Build history of the part. All positions in model axes, mm. A direction names the side the tool comes from. Round coordinates to 2 decimals unless told otherwise and drop trailing zeros. Loops run counter-clockwise (first coordinate to the right, second up) from the corner with the lowest first, then second, coordinate; pieces in that order, holes last. Notation, with made-up numbers: (86, 80.25) - (96, 80.25) arc R14 ccw to (96, 103.25) - close; hole circle Ø7 at (-30.75, 22). An arc over 180 degrees is marked (long way). One line per question, with ' | ' between items. Start each with the question number.
Autodesk Inventor part; units mm, degrees
ref_plane "YZ Plane" through (0, 0, 0) normal (1, 0, 0) x (0, 1, 0)
ref_plane "XZ Plane" through (0, 0, 0) normal (0, 1, 0) x (-1, 0, 0)
ref_plane "XY Plane" through (0, 0, 0) normal (0, 0, 1) x (1, 0, 0)
sketch "Sketch1" plane through (0, 0, 0) normal (0, 1, 0) x (-1, 0, 0)
  line L0 (22.352, 6.35) -> (-46.355, 6.35)
  line L1 (-46.355, 6.35) -> (-46.355, -6.35)
  line L2 (-46.355, -6.35) -> (22.352, -6.35)
  line L3 (22.352, -6.35) -> (22.352, 6.35)
  line L4 (-2.54, -2.54) -> (2.54, -2.54)
  line L5 (2.54, -2.54) -> (2.54, 2.54)
  line L6 (2.54, 2.54) -> (-2.54, 2.54)
  line L7 (-2.54, 2.54) -> (-2.54, -2.54)
  line L8 (-2.54, -2.54) -> (2.54, 2.54) construction
  line L9 (2.54, -2.54) -> (-2.54, 2.54) construction
  line L10 (-10.16, 2.54) -> (-15.24, 2.54)
  line L11 (-15.24, 2.54) -> (-15.24, -2.54)
  line L12 (-15.24, -2.54) -> (-10.16, -2.54)
  line L13 (-10.16, -2.54) -> (-10.16, 2.54)
  line L14 (-10.16, 2.54) -> (-15.24, -2.54) construction
  line L15 (-15.24, 2.54) -> (-10.16, -2.54) construction
  line L16 (-22.86, 2.54) -> (-27.94, 2.54)
  line L17 (-27.94, 2.54) -> (-27.94, -2.54)
  line L18 (-27.94, -2.54) -> (-22.86, -2.54)
  line L19 (-22.86, -2.54) -> (-22.86, 2.54)
  line L20 (-22.86, 2.54) -> (-27.94, -2.54) construction
  line L21 (-27.94, 2.54) -> (-22.86, -2.54) construction
  point P0 (0, 0)
  point P1 (-12.7, 0)
  point P2 (-25.4, 0)
  dimension "d0" = 68.707
  dimension "d1" = 12.7
  dimension "d2" = 5.08
  dimension "d3" = 5.08
  dimension "d4" = 5.08
  dimension "d5" = 5.08
  dimension "d6" = 12.7
  dimension "d7" = 12.7
  dimension "d8" = 6.35
  dimension "d9" = 22.352
  dimension "d37" = 5.08
  dimension "d38" = 5.08
extrude "Extrusion1" add sketch "Sketch1" along normal blind 2.286
sketch "Sketch2" plane through (0, 2.286, 0) normal (0, 1, 0) x (1, 0, 0)
  line L0 (-22.352, 6.35) -> (-22.352, -6.35)
  circle A0 centre (-16.002, 0) radius 4.191
  point P0 (0, 0)
  dimension "d12" = 6.35
  dimension "d13" = 8.382
extrude "Extrusion2" add sketch "Sketch2" along normal blind 5.207
sketch "Sketch3" plane through (-16.002, 7.493, 0) normal (0, 1, 0) x (1, 0, 0)
  circle A0 centre (0, 0) radius 3.2385
  point P0 (16.002, 0)
  dimension "d16" = 6.477
extrude "Extrusion3" cut sketch "Sketch3" against normal blind 0.7874
sketch "Sketch4" plane through (0, 0, 0) normal (0, -1, 0) x (1, 0, 0)
  circle A0 centre (-16.002, 0) radius 3.2385
  circle A1 centre (-16.002, 0) radius 3.2385
  point P0 (0, 0)
  dimension "d39" = 6.477
extrude "Extrusion4" cut sketch "Sketch4" against normal blind 0.7874
sketch "Sketch5" plane through (-16.002, 6.7056, 0) normal (0, 1, 0) x (1, 0, 0)
  circle A0 centre (0, 0) radius 2.7051
  point P0 (16.002, 0)
  dimension "d21" = 5.4102
extrude "Extrusion5" cut sketch "Sketch5" against normal through all
sketch "Sketch6" plane through (0, 2.286, 0) normal (0, 1, 0) x (1, 0, 0)
  line L0 (46.355, -6.35) -> (46.355, 6.35)
  circle A0 centre (40.005, 0) radius 4.191
  point P0 (0, 0)
  dimension "d24" = 6.35
  dimension "d25" = 8.382
extrude "Extrusion6" add sketch "Sketch6" along normal blind 5.207
sketch "Sketch7" plane through (40.005, 7.493, 0) normal (0, 1, 0) x (1, 0, 0)
  circle A0 centre (0, 0) radius 3.2385
  point P0 (-40.005, 0)
  dimension "d28" = 6.477
extrude "Extrusion7" cut sketch "Sketch7" against normal blind 0.7874
sketch "Sketch8" plane through (0, 0, 0) normal (0, -1, 0) x (1, 0, 0)
  circle A0 centre (40.005, 0) radius 3.2385
  circle A1 centre (40.005, 0) radius 3.2385
  point P0 (0, 0)
  dimension "d40" = 6.477
extrude "Extrusion8" cut sketch "Sketch8" against normal blind 0.7874
sketch "Sketch9" plane through (40.005, 6.7056, 0) normal (0, 1, 0) x (1, 0, 0)
  circle A0 centre (0, 0) radius 2.7051
  point P0 (-40.005, 0)
  dimension "d33" = 5.4102
extrude "Extrusion9" cut sketch "Sketch9" against normal through all
fillet "Fillet1" radius 6.35 4 edges at (46.355, 1.143, 6.35) (46.355, 1.143, -6.35) (-22.352, 1.143, 6.35) (-22.352, 1.143, -6.35)
sketch "Sketch12" plane through (-16.002, 7.493, 0) normal (0, 1, 0) x (1, 0, 0)
  circle A0 centre (0, 0) radius 4.191
  line L0 (0, 0) -> (4.0259, 0) construction
  line L1 (0, 0) -> (4.0259, 0) construction
  circle A1 centre (0, 0) radius 3.2385
  line L2 (-3.1893, 0.5624) -> (-4.1273, 0.7278)
  line L3 (-3.1893, -0.5624) -> (-4.1273, -0.7278)
  arc A2 (-3.1893, 0.5624) -> (-3.1893, -0.5624) centre (0, 0) ccw
  arc A3 (-4.1273, 0.7278) -> (-4.1273, -0.7278) centre (0, 0) ccw
  point P0 (16.002, 0)
  point P1 (-2.9392, 0.5183)
extrude "Extrusion11" cut sketch "Sketch12" against normal blind 0.762 contours L2 A1 L3 A0 picked at (-3.8669, 0.0628)
properties part number "VexLegoMountThick3"
1) Tool access for faces 1 (the cylindrical face through (-13.01, 7.1, 1.24)), 2 (the flat face through (0, 1, -2.54)), 3 (the flat face through (-13, 7.493, 2)): list every direction of +Z, -Z, +X, -X, +Y, -Y with a clear straight run to the whole face (end or side of a thin tool).
2) Saw through at D-D on x = 20.5. Write the cut outline in (y, z).
3) Saw through at C-C on y = 1.5. State how many separate pieces and enclosed holes the cut face has, and give its area (3 significant figures).
4) Saw through at A-A on x = -1. Write the cut outline in (y, z).
5) Wall check: line 1 (X direction, y = 2.85, z = 0); line 2 (X direction, y = 2.25, z = 1.25); line 3 (X direction, y = 7.25, z = 1). Give the ranges that are in metal, low to high. Write a range as [from, to].
6) Drop flat-ended pins along their axis: pin 1 (0.7 mm diameter, centred on y = 1.5, z = 1, fed in from +X); pin 2 (7 mm diameter, centred on x = 38.5, z = 1, fed in from +Y); pin 3 (6 mm diameter, centred on x = 40.005, z = 0, fed in from +Y); pin 4 (1.5 mm diameter, centred on y = 6, z = 4, fed in from +X). Give the stop position or say it passes through.
7) Saw through at B-B on y = 4.75. Write the cut outline in (x, z) (3 decimals).
Answer key:
1) face 1: +Y | face 2: +Y, -Y | face 3: +Z, -Z, +X, -X, +Y
2) outline: (0, -6.35) - (2.29, -6.35) - (2.29, 6.35) - (0, 6.35) - close
3) separate pieces: 1 | enclosed holes: 5 | area: 715 mm²
4) outline: (0, -6.35) - (2.29, -6.35) - (2.29, -2.54) - (0, -2.54) - close; (0, 2.54) - (2.29, 2.54) - (2.29, 6.35) - (0, 6.35) - close
5) line 1: [-20.19, -18.71], [-13.3, -11.81], [35.81, 37.3], [42.71, 44.2] | line 2: [-22.23, -18.4], [-13.6, -2.54], [2.54, 10.16], [15.24, 22.86], [27.94, 37.61], [42.4, 46.23] | line 3: [-20.07, -19.08], [-12.92, -11.93], [35.94, 36.92], [43.09, 44.07]
6) pin 1: x = 46.32 | pin 2: y = 7.49 | pin 3: y = 6.71 | pin 4: x = 42.65
7) outline: circle Ø8.382 at (-16.002, 0); circle Ø8.382 at (40.005, 0); hole circle Ø5.41 at (-16.002, 0); hole circle Ø5.41 at (40.005, 0)
